Check sheet for the drawn part. Datum: minimum x, y, z corner. Units: mm. Coordinates: 2 decimals unless noted, no trailing zeros. Order: outer loops, then holes, each group sorted by start corner. A loop starts at its lowest first (then second) coordinate and runs counter-clockwise, first axis right, second up.
1. Gauge pin test, flat ends, axial feed: pin 1 Ø5 at (x, y) = (74, 13) entering from -Z; pin 2 Ø1.5 at (y, z) = (5.5, 22) entering from -X; pin 3 Ø3 at (y, z) = (15, 67) entering from -X. Record the tip position at first contact, or that the pin passes through.
2. Thickness scan on line 1 (Z direction, x = 44.5, y = 14.5); line 2 (Z direction, x = 44, y = 18.25); line 3 (X direction, y = 8, z = 20.5). Record the ranges inside material, lowest first.
3. Cross-section at A-A (y = 12.5). Enter the section's corners in (x, z).
4. Cross-section at B-B (z = 40.5). Enter the section's corners in (x, y).
5. Draft check along Z on the marked faces 1, 2, 3 and 4. Enter one of: released by +Z, released by -Z, zero draft, split by the parting line, or undercut.
6. Cross-section at C-C (x = 72). Enter the section's corners in (y, z) (1 decimal), then the cut area to 3 significant figures.
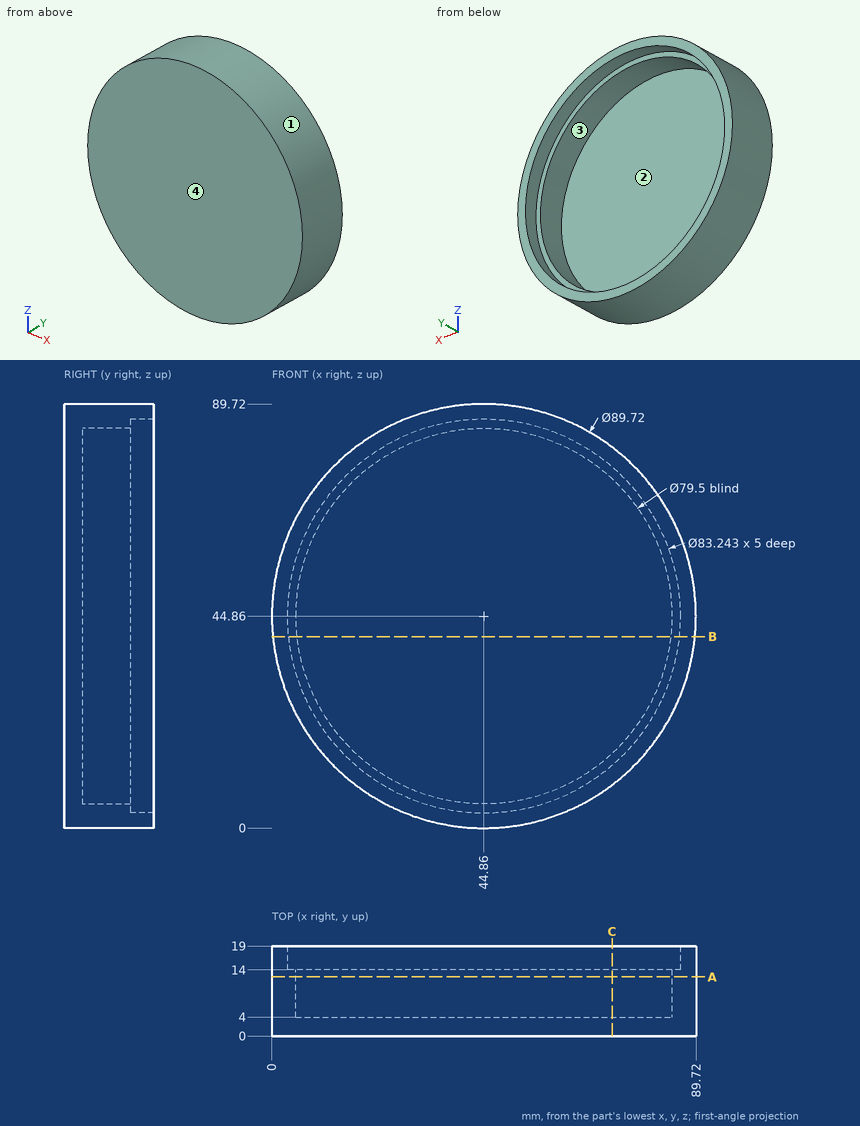
Data:
1. pin 1: stops at z = 8.77
1. pin 2: stops at x = 5.83
1. pin 3: stops at x = 5.03
2. line 1: z = 0 to 3.24, 86.48 to 89.72
2. line 2: z = 0.01 to 3.25, 86.47 to 89.71
2. line 3: x = 7.19 to 13.45, 76.27 to 82.53
3. outline: circle Ø89.72 at (44.86, 44.86); hole circle Ø79.5 at (44.86, 44.86)
4. outline: (0.21, 0) - (89.51, 0) - (89.51, 19) - (86.25, 19) - (86.25, 14) - (84.37, 14) - (84.37, 4) - (5.35, 4) - (5.35, 14) - (3.47, 14) - (3.47, 19) - (0.21, 19) - close
5. face 1: split by the parting line
5. face 2: undercut
5. face 3: undercut
5. face 4: zero draft
6. outline: (0, 9.1) - (19, 9.1) - (19, 13.3) - (14, 13.3) - (14, 15.8) - (4, 15.8) - (4, 73.9) - (14, 73.9) - (14, 76.4) - (19, 76.4) - (19, 80.6) - (0, 80.6) - close
6. area: 461 mm2
